The figure shows three views and two pictorial views of one solid part (mm, origin at its lowest corner). Answer the questions. A direction names the side the tool comes from. Coordinates: 2 decimals unless noted, no trailing zeros. Loops run counter-clockwise (first coordinate to the right, second up) from the corner with the lowest first, then second, coordinate; pieces in that order, holes last. Notation, with made-up numbers: M 65,56 L 98,56 A20 ccw 98,63 Z; hole C 3,-11 d5. An arc over 180 degrees is marked long. Answer as a JSON object with one key per item and string values. Group by question number.
1. For the marked faces 1, 2 and 3, determine the directions among +Z, -Z, +X, -X, +Y, -Y from which every point of the face is accessible in a straight line to the end or side of a thin tool.
2. Straight lines are drawn through the part: L1, parallel to Z at x = 49, y = 32; L2, parallel to Y at x = 48, z = 174.5; L3, parallel to Z at x = 41.5, y = 25.5 (1 decimal). For each, find the intervals that lie inside material, in ascending order.
3. A cutting plane is placed at B-B on y = 42. Give the vertices of the cut face in (x, z) (1 decimal), and give its area (3 significant figures).
4. Determine the mould class of the marked faces 4, 5 and 6 for opening direction Z: released by +Z, released by -Z, zero draft, split by the parting line, or undercut.
5. A cutting plane is placed at C-C on z = 139. Give the vertices of the cut face in (x, y).
6. A cutting plane is placed at D-D on y = 15.5. Give the vertices of the cut face in (x, z), and give its area (3 significant figures).
7. Given pin 1 (6 mm diameter, centred on x = 28, y = 47, fed in from +Z); pin 2 (17.5 mm diameter, centred on y = 25.5, z = 183, fed in from -X); pin 3 (21 mm diameter, centred on x = 38, z = 185.5, fed in from +Y); pin 4 (5.5 mm diameter, centred on y = 28.35, z = 185.9, fed in from -X), each flat-ended and moving along its own axis, determine where each tip first touches the part or whether it passes through.
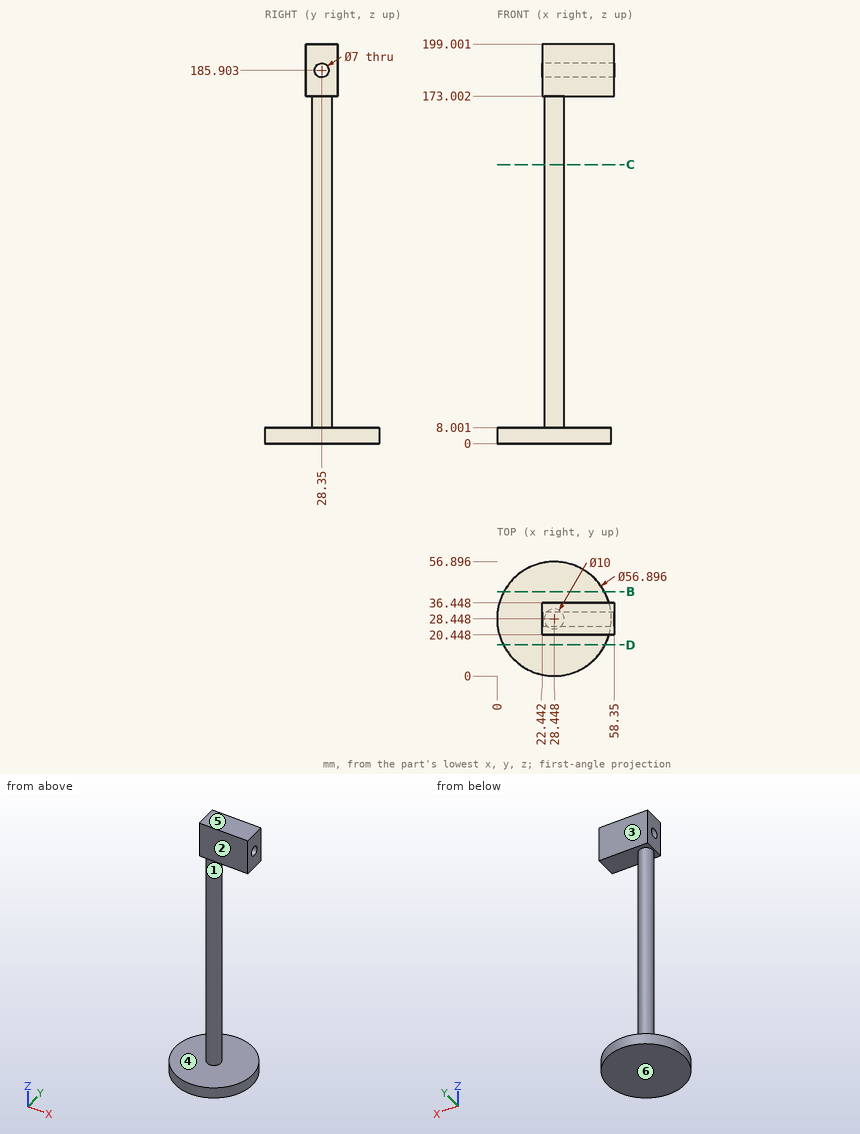
From the geometry:
{
 "1": {"face 1": "none", "face 2": "+Z, +X, -X, -Y", "face 3": "+Z, +X, -X, +Y"},
 "2": {"L1": "z = 0 to 8, 173 to 199", "L2": "y = 20.45 to 36.45", "L3": "z = 0 to 8, 173 to 183.9, 187.9 to 199"},
 "3": {"outline": "M 3.4,0 L 53.5,0 L 53.5,8 L 3.4,8 Z", "area": "400 mm²"},
 "4": {"face 4": "undercut", "face 5": "released by +Z", "face 6": "released by -Z"},
 "5": {"outline": "C 28.45,28.45 d10"},
 "6": {"outline": "M 3.12,0 L 53.78,0 L 53.78,8 L 3.12,8 Z", "area": "405 mm²"},
 "7": {"pin 1": "stops at z = 8", "pin 2": "stops at x = 22.44", "pin 3": "stops at y = 36.45", "pin 4": "passes through"}
}
